```python
from build123d import *

# Parameters (mm, degrees)
PAD_DEPTH       = 11
SKETCH001_R     = 25
SKETCH001_R_2   = 15
PAD001_DEPTH    = 3
SKETCH002_R     = 7
PAD002_DEPTH    = 35
SKETCH003_R     = 30
PAD003_DEPTH    = 58
PAD004_DEPTH    = 22
SKETCH006_R     = 19.05
POCKET_DEPTH    = 4
SKETCH007_R     = 2.25
HOLE_DEPTH      = 6.648064
HOLE_TIPS_R     = 2.25
SKETCH008_R     = 4
POCKET001_DEPTH = 27
SKETCH009_R     = 2.75
HOLE001_DEPTH   = 23.347633
HOLE001_TIPS_R  = 2.75


with BuildPart() as part:
    # Sketch → Pad (new body)
    with BuildSketch(Plane.XZ):
        with BuildLine():
            Line((-25.69533, 30), (25.69533, 30))
            ThreePointArc((30, 25.69533), (27.930718, 27.930718), (25.69533, 30))
            Line((30, 25.69533), (30, -25.69533))
            ThreePointArc((25.69533, -30), (27.930718, -27.930718), (30, -25.69533))
            Line((25.69533, -30), (-25.69533, -30))
            ThreePointArc((-30, -25.69533), (-27.930718, -27.930718), (-25.69533, -30))
            Line((-30, -25.69533), (-30, 25.69533))
            ThreePointArc((-25.69533, 30), (-27.930718, 27.930718), (-30, 25.69533))
        make_face()
    extrude(amount=PAD_DEPTH)

    # Sketch001 (on Face10 of Pad) → Pad001 (join)
    with BuildSketch(Plane.XZ.offset(11)):
        Circle(SKETCH001_R)
        Circle(SKETCH001_R_2, mode=Mode.SUBTRACT)
    extrude(amount=PAD001_DEPTH)

    # Sketch002 (on Face14 of Pad001) → Pad002 (join)
    with BuildSketch(Plane.XZ.offset(11)):
        Circle(SKETCH002_R)
    extrude(amount=PAD002_DEPTH)

    # Sketch003 (on Face4 of Pad002) → Pad003 (join)
    with BuildSketch(Plane(origin=(0, 0, 0), x_dir=(1, 0, 0), z_dir=(0, 1, 0))):
        Circle(SKETCH003_R)
    extrude(amount=PAD003_DEPTH)

    # Sketch004 (on Face16 of Pad003) → Pad004 (join)
    with BuildSketch(Plane(origin=(0, 58, 0), x_dir=(1, 0, 0), z_dir=(0, 1, 0))):
        with BuildLine():
            ThreePointArc((-30, -25.69533), (-27.930718, -27.930718), (-25.69533, -30))
            Line((25.69533, -30), (-25.69533, -30))
            ThreePointArc((25.69533, -30), (27.930718, -27.930718), (30, -25.69533))
            Line((30, 25.69533), (30, -25.69533))
            ThreePointArc((30, 25.69533), (27.930718, 27.930718), (25.69533, 30))
            Line((-25.69533, 30), (25.69533, 30))
            ThreePointArc((-25.69533, 30), (-27.930718, 27.930718), (-30, 25.69533))
            Line((-30, -25.69533), (-30, 25.69533))
        make_face()
    extrude(amount=PAD004_DEPTH)

    # Sketch005 → Groove (revolve, cut)
    with BuildSketch(Plane.YZ):
        Polygon((80, 68.105118), (58, 30), (58, 68.105118), align=None)
    revolve(axis=Axis((0, 0, 0), (0, 1, 0)), mode=Mode.SUBTRACT)

    # Sketch006 (on Face30 of Groove) → Pocket (cut)
    with BuildSketch(Plane(origin=(0, 80, 0), x_dir=(1, 0, 0), z_dir=(0, 1, 0))):
        Circle(SKETCH006_R)
    extrude(amount=-POCKET_DEPTH, mode=Mode.SUBTRACT)

    # Sketch007 (on Face30 of Pocket) → Hole (cut)
    with BuildSketch(Plane(origin=(0, 80, 0), x_dir=(1, 0, 0), z_dir=(0, 1, 0))):
        with Locations((-23.55, -23.55)):
            Circle(SKETCH007_R)
        with Locations((23.55, -23.55)):
            Circle(SKETCH007_R)
        with Locations((-23.55, 23.55)):
            Circle(SKETCH007_R)
        with Locations((23.55, 23.55)):
            Circle(SKETCH007_R)
    extrude(amount=-HOLE_DEPTH, mode=Mode.SUBTRACT)

    # Hole tips → Hole tip 1 section 0
    with BuildSketch(Plane(origin=(0, 73.351936, 0), x_dir=(1, 0, 0), z_dir=(0, 1, 0)), mode=Mode.PRIVATE) as hole_tip_1_s0:
        with Locations((-23.55, -23.55)):
            Circle(HOLE_TIPS_R)
    loft([hole_tip_1_s0.sketch, Vertex(-23.55, 72, 23.55)], mode=Mode.SUBTRACT)

    # Hole tips → Hole tip 2 section 0
    with BuildSketch(Plane(origin=(0, 73.351936, 0), x_dir=(1, 0, 0), z_dir=(0, 1, 0)), mode=Mode.PRIVATE) as hole_tip_2_s0:
        with Locations((23.55, -23.55)):
            Circle(HOLE_TIPS_R)
    loft([hole_tip_2_s0.sketch, Vertex(23.55, 72, 23.55)], mode=Mode.SUBTRACT)

    # Hole tips → Hole tip 3 section 0
    with BuildSketch(Plane(origin=(0, 73.351936, 0), x_dir=(1, 0, 0), z_dir=(0, 1, 0)), mode=Mode.PRIVATE) as hole_tip_3_s0:
        with Locations((-23.55, 23.55)):
            Circle(HOLE_TIPS_R)
    loft([hole_tip_3_s0.sketch, Vertex(-23.55, 72, -23.55)], mode=Mode.SUBTRACT)

    # Hole tips → Hole tip 4 section 0
    with BuildSketch(Plane(origin=(0, 73.351936, 0), x_dir=(1, 0, 0), z_dir=(0, 1, 0)), mode=Mode.PRIVATE) as hole_tip_4_s0:
        with Locations((23.55, 23.55)):
            Circle(HOLE_TIPS_R)
    loft([hole_tip_4_s0.sketch, Vertex(23.55, 72, -23.55)], mode=Mode.SUBTRACT)

    # Sketch008 (on Face41 of Hole) → Pocket001 (cut)
    with BuildSketch(Plane(origin=(0, 76, 0), x_dir=(1, 0, 0), z_dir=(0, 1, 0))):
        Circle(SKETCH008_R)
    extrude(amount=-POCKET001_DEPTH, mode=Mode.SUBTRACT)

    # Sketch009 (on Face6 of Pocket001) → Hole001 (cut)
    with BuildSketch(Plane.XZ.offset(11)):
        with Locations((-24.748737, 24.748737)):
            Circle(SKETCH009_R)
        with Locations((24.748737, 24.748737)):
            Circle(SKETCH009_R)
        with Locations((24.748737, -24.748737)):
            Circle(SKETCH009_R)
        with Locations((-24.748737, -24.748737)):
            Circle(SKETCH009_R)
    extrude(amount=-HOLE001_DEPTH, mode=Mode.SUBTRACT)

    # Hole001 tips → Hole001 tip 1 section 0
    with BuildSketch(Plane.XZ.offset(-12.347633), mode=Mode.PRIVATE) as hole001_tip_1_s0:
        with Locations((-24.748737, 24.748737)):
            Circle(HOLE001_TIPS_R)
    loft([hole001_tip_1_s0.sketch, Vertex(-24.748737, 14, 24.748737)], mode=Mode.SUBTRACT)

    # Hole001 tips → Hole001 tip 2 section 0
    with BuildSketch(Plane.XZ.offset(-12.347633), mode=Mode.PRIVATE) as hole001_tip_2_s0:
        with Locations((24.748737, 24.748737)):
            Circle(HOLE001_TIPS_R)
    loft([hole001_tip_2_s0.sketch, Vertex(24.748737, 14, 24.748737)], mode=Mode.SUBTRACT)

    # Hole001 tips → Hole001 tip 3 section 0
    with BuildSketch(Plane.XZ.offset(-12.347633), mode=Mode.PRIVATE) as hole001_tip_3_s0:
        with Locations((24.748737, -24.748737)):
            Circle(HOLE001_TIPS_R)
    loft([hole001_tip_3_s0.sketch, Vertex(24.748737, 14, -24.748737)], mode=Mode.SUBTRACT)

    # Hole001 tips → Hole001 tip 4 section 0
    with BuildSketch(Plane.XZ.offset(-12.347633), mode=Mode.PRIVATE) as hole001_tip_4_s0:
        with Locations((-24.748737, -24.748737)):
            Circle(HOLE001_TIPS_R)
    loft([hole001_tip_4_s0.sketch, Vertex(-24.748737, 14, -24.748737)], mode=Mode.SUBTRACT)


solid = part.part
```
Input: part model. Units: mm. Frame: model coordinates. A direction names the side the tool comes from. Round coordinates to 2 decimals unless told otherwise and drop trailing zeros. Loops run counter-clockwise (first coordinate to the right, second up) from the corner with the lowest first, then second, coordinate; pieces in that order, holes last. Notation, with made-up numbers: (33.25, 60.25) - (44.25, 60.25) arc R18 cw to (44.25, 94.25) - close; hole circle Ø4 at (40.25, -19.75). An arc over 180 degrees is marked (long way). One line per item, written item: value. Start each with the question number.
(1) Section B-B, the plane y = -24. Return loops of the section in (x, z).
(2) Contact query for flat-ended pins moving along their axis: P1, Ø10, axis at y = 53.5, z = 23.5, coming from the +X side; P2, Ø6, axis at x = 23.55, z = 23.55, coming from the +Y side; P3, Ø6.5, axis at x = 1, z = 0.5, coming from the +Y side; P4, Ø1.5, axis at x = 23, z = 3, coming from the -Y side. Output: stop coordinate, or through.
(3) Draft query along X for faces 6 (the cylindrical face through (27.9, 71.63, 27.96)), 7 (the conical face through (-23.218, 72.216, -23.412)), 8 (the cylindrical face through (-27.96, 71.63, 27.9)). Return one class per face: +X half, -X half, draft (parallel to the pull), parting line (faces both ways), or undercut.
(4) Ray query, line 1 (X direction, y = 78, z = 23.55); line 2 (Z direction, x = -23, y = 77); line 3 (X direction, y = 78.2, z = 0). Return the intervals inside material, ascending. Write a range as [from, to].
(5) Section A-A, the plane y = 24.5. Return loops of the section in (x, z), plus the area to 3 significant figures.
(6) Access query for faces 1 (the cylindrical face through (-25.345, -5.577, 22.064)), 2 (the flat face through (-14, 80, -14)), 3 (the flat face through (23, 0, 22)), 4 (the cylindrical face through (-24.038, 76.723, -21.354)), 5 (the flat face through (-30, -5, 0)). Directions: +Z, -Z, +X, -X, +Y, -Y. A direction counts if a zero-diameter tool reaches every point of the face in a straight line with its end or side. Return the directions, or none.
Results below:
1. outline: circle Ø14 at (0, 0)
2. P1: x = 23.62
2. P2: y = 80
2. P3: y = 76
2. P4: y = -14
3. face 6: +X half
3. face 7: undercut
3. face 8: -X half
4. line 1: [-30, -25.8], [-21.3, 21.3], [25.8, 30]
4. line 2: [-30, -25.73], [-21.37, 21.37], [25.73, 30]
4. line 3: [-30, -19.05], [19.05, 30]
5. outline: circle Ø60 at (0, 0)
5. area: 2,830 mm^2
6. face 1: -Y
6. face 2: +Z, -Z, +X, -X, +Y
6. face 3: +Z, +X
6. face 4: +Y
6. face 5: +Z, -Z, -X, +Y, -Y
